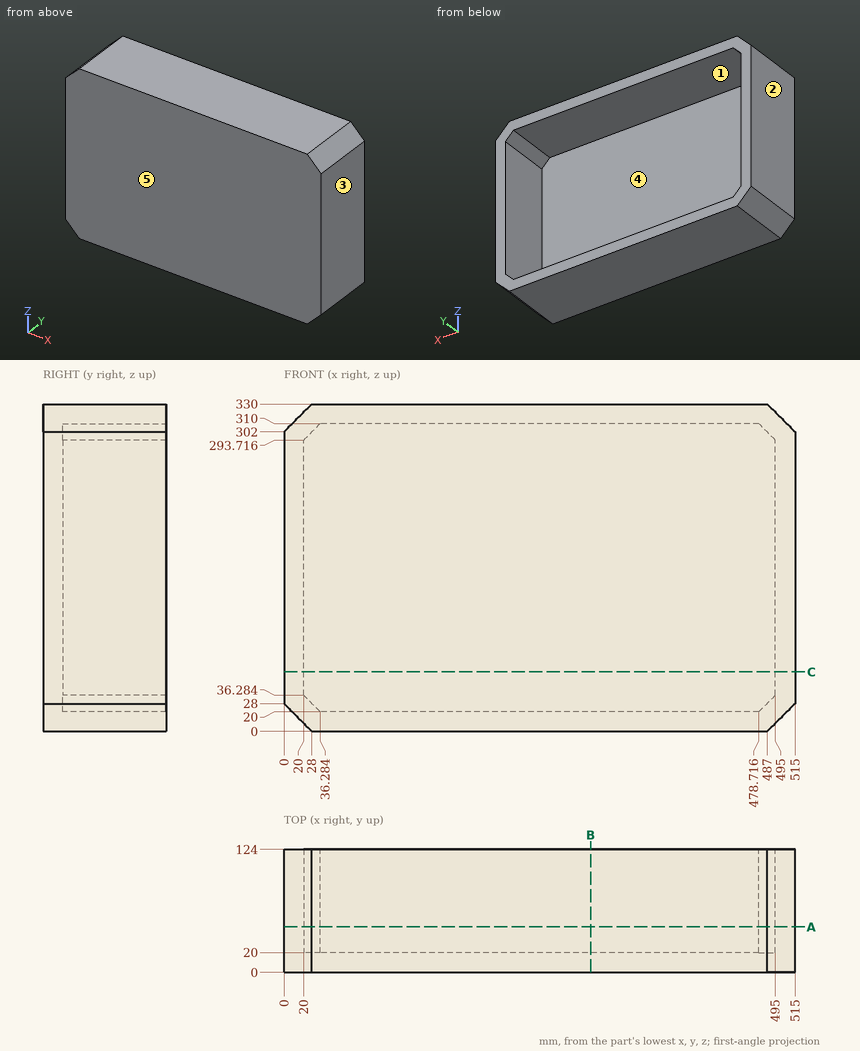
Drawing for the job (mm, zero at the part's lowest x, y, z). A direction names the side the tool comes from. Coordinates: 2 decimals unless noted, no trailing zeros. Loops run counter-clockwise (first coordinate to the right, second up) from the corner with the lowest first, then second, coordinate; pieces in that order, holes last. Notation, with made-up numbers: (74.25, -13.5) - (96.25, -13.5) arc R29 cw to (96.25, 9.5) - close; hole circle Ø3 at (72.25, -25.5). An arc over 180 degrees is marked (long way). Use CSV: the item, a comma, the result in double quotes. Start each with the question number.
Q1. Two-plate mould, pull along X, no slides. Class the marked faces 3, 4 and 5: +X half, -X half, draft (parallel to the pull), parting line (faces both ways), or undercut.
Q2. Cut at C-C, the plane z = 60. List the corners of the cut face in (x, y).
Q3. Cut at A-A, the plane y = 46. List the corners of the cut face in (x, z).
Q4. Drop a flat-ended pin along its axis: P1, Ø5, axis at x = 143.5, z = 147.5, coming from the +Y side. Give the stop position or say it passes through.
Q5. 3-axis set-ups, long thin cutter, end or side, ignore diameter. For the marked faces 1 and 2: which of +Z, -Z, +X, -X, +Y, -Y reach the whole face in a straight line?
Q6. Probe probe 1 along X at (y, z) = (40.5, 63); probe 2 along Z at (x, y) = (352, 22); probe 3 along Y at (x, z) = (21, 68). List the from-to ranges inside material, lowest first. Write a range as from..to.
Q7. Cut at B-B, the plane x = 309. List the corners of the cut face in (y, z).
Here are the results:
1,face 3,"+X half"
1,face 4,"undercut"
1,face 5,"draft"
2,outline,"(0, 0) - (515, 0) - (515, 124) - (495, 124) - (495, 20) - (20, 20) - (20, 124) - (0, 124) - close"
3,outline,"(0, 28) - (28, 0) - (487, 0) - (515, 28) - (515, 302) - (487, 330) - (28, 330) - (0, 302) - close; hole (20, 36.28) - (36.28, 20) - (478.72, 20) - (495, 36.28) - (495, 293.72) - (478.72, 310) - (36.28, 310) - (20, 293.72) - close"
4,P1,"y = 20"
5,face 1,"+Y"
5,face 2,"+Z, -Z, -X, +Y, -Y"
6,probe 1,"0..20, 495..515"
6,probe 2,"0..20, 310..330"
6,probe 3,"0..20"
7,outline,"(0, 0) - (124, 0) - (124, 20) - (20, 20) - (20, 310) - (124, 310) - (124, 330) - (0, 330) - close"
